Build history of the part. All positions in model axes, mm. Face numbers are marked on the shaded views. A direction names the side the tool comes from. Give positions to 0.01 mm unless a question says otherwise; leave off trailing zeros. Order: outer loops, then holes, each group sorted by start corner. A loop starts at its lowest first (then second) coordinate and runs counter-clockwise, first axis right, second up. Notation, with made-up numbers: (59.5, -16) -> (72.5, -16) arc R24 ccw to (72.5, 10) -> close; hole circle Ø2 at (55, 57.5). An arc over 180 degrees is marked (long way). One line per item, written item: value. Start each with the question number.
(1) Saw through at B-B on y = -36. Give the cut face in (x, z), plus the area to 3 significant figures.
(2) Saw through at D-D on x = 11.5. Give the cut face in (y, z).
(3) Two-plate mould, pull along Y, no slides. Class the marked faces 1, 2, 3 and 4: +Y half, -Y half, draft (parallel to the pull), parting line (faces both ways), or undercut.
(4) Probe line 1 (Z direction, x = 40.5, y = -6.5); line 2 (Y direction, x = 21.5, z = 35); line 3 (Y direction, x = 23, z = 33). List the from-to ranges inside material, lowest first.
(5) Which spindle directions (+Z, -Z, +X, -X, +Y, -Y) get a long thin tool onto all of the face, cutting with end or side? Do the marked faces 5 and 6. Say none if no direction does.
(6) Saw through at C-C on z = 17.5. Give the cut face in (x, y), plus the area to 3 significant figures.
(7) Pin check, flat tips, straight feed: pin 1 (12 mm diameter, centred on x = 13.5, y = -23, fed in from +Z); pin 2 (3 mm diameter, centred on x = 32.5, z = 17, fed in from -Y); pin 3 (8 mm diameter, centred on y = -31.5, z = 11, fed in from +X). Stop position of each tip, or through.
(8) Saw through at A-A on x = 19.5. Give the cut face in (y, z).
```python
from build123d import *

# Parameters (mm, degrees)
SKETCH1_R           = 42
BOSS_EXTRUDE1_DEPTH = 41
CUT_EXTRUDE1_DEPTH  = 73.173402303
SKETCH3_R           = 7.7
CUT_EXTRUDE2_DEPTH  = 73.173402303
SKETCH4_W           = 0.6
SKETCH4_H           = 34.211954595
SKETCH4_W_2         = 35.741543893
SKETCH4_H_2         = 0.6
CUT_EXTRUDE3_DEPTH  = 73.173402476
CUT_EXTRUDE4_DEPTH  = 19
CUT_EXTRUDE6_START  = -19
CUT_EXTRUDE6_DEPTH  = 19
FILLET1_R           = 1.5


with BuildPart() as part:
    # Sketch1 → Boss-Extrude1 (new body)
    with BuildSketch(Plane.XY):
        Circle(SKETCH1_R)
    extrude(amount=BOSS_EXTRUDE1_DEPTH)

    # Sketch2 → Cut-Extrude1 (cut, through all)
    with BuildSketch(Plane.XY.offset(41)):
        with BuildLine():
            Line((0, 0), (42, 0))
            ThreePointArc((42, 0), (-29.69848481, 29.69848481), (0, -42))
            Line((0, -42), (0, 0))
        make_face()
    extrude(amount=-CUT_EXTRUDE1_DEPTH, mode=Mode.SUBTRACT)

    # Sketch3 → Cut-Extrude2 (cut, through all)
    with BuildSketch(Plane(origin=(0, 0, 0), x_dir=(1, 0, 0), z_dir=(0, 1, 0))):
        Circle(SKETCH3_R)
    extrude(amount=-CUT_EXTRUDE2_DEPTH, mode=Mode.SUBTRACT)

    # Sketch4 → Cut-Extrude3 (cut, through all)
    with BuildSketch(Plane(origin=(0, 0, 0), x_dir=(1, 0, 0), z_dir=(0, 1, 0))):
        with Locations((0.3, -23.894022702)):
            Rectangle(SKETCH4_W, SKETCH4_H)
        with Locations((24.129228054, -0.3)):
            Rectangle(SKETCH4_W_2, SKETCH4_H_2)
    extrude(amount=-CUT_EXTRUDE3_DEPTH, mode=Mode.SUBTRACT)

    # Sketch5 → Cut-Extrude4 (cut)
    with BuildSketch(Plane.XY.offset(41)):
        Polygon((36.041125497, -15.470562748), (33.212698372, -12.642135624), (13.413708499, -32.441125497), (16.242135624, -35.269552622), align=None)
        Polygon((33.919805153, -3.449747468), (31.712698372, -5.656854249), (6.256854249, -31.112698372), (2.1, -35.269552622), (6.342640687, -39.512193309), (13.413708499, -32.441125497), (33.212698372, -12.642135624), (38.162445841, -7.692388155), align=None)
    extrude(amount=-CUT_EXTRUDE4_DEPTH, mode=Mode.SUBTRACT)

    # Sketch6 → Cut-Extrude6 (cut)
    with BuildSketch(Plane.XY.offset(41).offset(CUT_EXTRUDE6_START)):
        with BuildLine():
            Line((28.970057685, -8.399494937), (6.327564928, -31.041987694))
            Line((6.327564928, -31.041987694), (0.670710678, -25.385133445))
            Line((0.670710678, -25.385133445), (26.055844123, 0))
            Line((26.055844123, 0), (42, 0))
            ThreePointArc((42, 0), (41.025156816, -8.996471987), (38.145880561, -17.575317813))
            Line((38.145880561, -17.575317813), (33.212698372, -12.642135624))
            Line((33.212698372, -12.642135624), (28.970057685, -8.399494937))
        make_face()
    extrude(amount=CUT_EXTRUDE6_DEPTH, mode=Mode.SUBTRACT)

    # Fillet1
    fillet1_edges = [part.edges().sort_by_distance(p)[0] for p in [
        (6.327564928, -31.041987694, 31.5),
        (26.055844123, 0, 31.5),
        (38.145880561, -17.575317813, 31.5),
        (36.041125497, -15.470562748, 31.5),
        (13.413708499, -32.441125497, 31.5),
    ]]
    fillet(fillet1_edges, radius=FILLET1_R)


solid = part.part
```
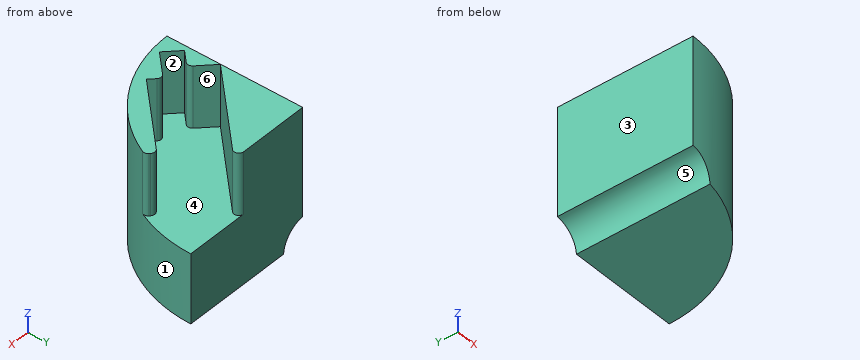
Results below:
1. outline: (0.6, 7.68) arc R7.7 cw to (7.68, 0.6) -> (21.63, 0.6) -> (21.63, 41) -> (9.85, 41) -> (9.85, 22) -> (2.83, 22) -> (2.83, 41) -> (0.6, 41) -> close
1. area: 679 mm²
2. outline: (-40.39, 0.6) -> (0, 0.6) -> (0, 41) -> (-14.56, 41) -> (-14.56, 22) -> (-34.35, 22) -> (-34.35, 41) -> (-40.39, 41) -> close
3. face 1: -Y half
3. face 2: undercut
3. face 3: draft
3. face 4: undercut
4. line 1: z = 0.6 to 22
4. line 2: y = -36.08 to -30.01, -4.56 to 0
4. line 3: y = -35.14 to -28.51, -3.06 to -0.11
5. face 5: -Z, -X, +Y, -Y
5. face 6: +Z
6. outline: (0.6, -42) arc R42 ccw to (42, 0) -> (0.6, 0) -> close
6. area: 1,360 mm²
7. pin 1: stops at z = 22
7. pin 2: stops at y = -28.34
7. pin 3: stops at x = 31.75
8. outline: (-37.2, 0.6) -> (0, 0.6) -> (0, 41) -> (-6.56, 41) -> (-6.56, 22) -> (-32.01, 22) -> (-32.01, 41) -> (-37.2, 41) -> close
